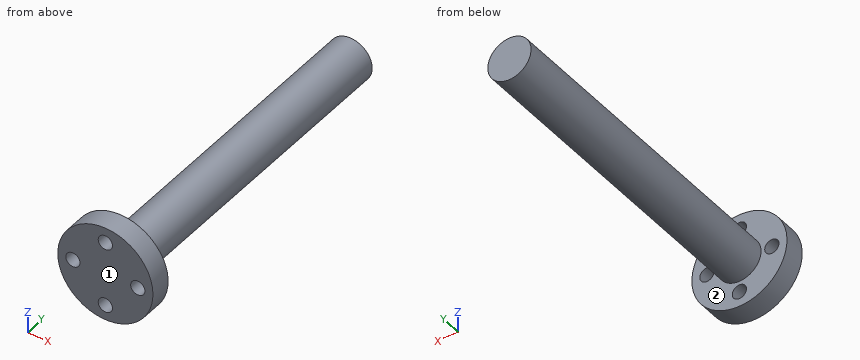
```python
from build123d import *

# Parameters (mm, degrees)
SKETCH1_R                                 = 10
OUTPUT_SHAFT_20MM_DEPTH                   = 161
SKETCH2_R                                 = 22
SKETCH2_R_2                               = 3.3
OUTPUT_LOWER_FLANGE_WITH_BOLT_HOLES_DEPTH = 10


with BuildPart() as part:
    # Sketch1 → Output_Shaft_20mm (new body)
    with BuildSketch(Plane(origin=(0, 0, 0), x_dir=(1, 0, 0), z_dir=(0, 1, 0))):
        with Locations(Location((0, 0, 0), (0, 0, 270))):
            Circle(SKETCH1_R)
    extrude(amount=OUTPUT_SHAFT_20MM_DEPTH)

    # Sketch2 → Output_Lower_Flange_With_Bolt_Holes (add)
    with BuildSketch(Plane(origin=(0, 0, 0), x_dir=(1, 0, 0), z_dir=(0, 1, 0))):
        with Locations(Location((0, 0, 0), (0, 0, 270))):
            Circle(SKETCH2_R)
        with Locations(Location((-15, 0, 0), (0, 0, 270))):
            Circle(SKETCH2_R_2, mode=Mode.SUBTRACT)
        with Locations(Location((15, 0, 0), (0, 0, 270))):
            Circle(SKETCH2_R_2, mode=Mode.SUBTRACT)
        with Locations(Location((0, -15, 0), (0, 0, 270))):
            Circle(SKETCH2_R_2, mode=Mode.SUBTRACT)
        with Locations(Location((0, 15, 0), (0, 0, 270))):
            Circle(SKETCH2_R_2, mode=Mode.SUBTRACT)
    extrude(amount=OUTPUT_LOWER_FLANGE_WITH_BOLT_HOLES_DEPTH)


solid = part.part
```
Check sheet for the modelled part. Datum: model origin and axes. Units: mm. Face numbers are marked on the shaded views. A direction names the side the tool comes from. Coordinates: 2 decimals unless noted, no trailing zeros. Order: outer loops, then holes, each group sorted by start corner. A loop starts at its lowest first (then second) coordinate and runs counter-clockwise, first axis right, second up. Notation, with made-up numbers: (15.25, 38.5) -> (53.25, 38.5) arc R32 cw to (53.25, 67.5) -> close; hole circle Ø4 at (26, 33.25). An arc over 180 degrees is marked (long way). Write each question's results on one line, items separated by ' | '. Start each with the question number.
1) Section check A-A (z = 0). Enter the section's corners in (x, y), and give its area (3 significant figures).
2) Section check C-C (x = 15). Enter the section's corners in (y, z).
3) Section check B-B (z = -15). Enter the section's corners in (x, y), and give its area (3 significant figures).
4) Set-up check for the marked faces 1 and 2: record each of +Z, -Z, +X, -X, +Y, -Y from which the full face is reachable in a straight line by a thin tool's end or side.
5) Material ranges on line 1 along X through (y, z) = (7, 0); line 2 along Y through (x, z) = (-20, -2.5); line 3 along Z through (x, y) = (-4, 41), recorded low to high.
6) Depth check by flat-ended pin: pin 1 (6 mm diameter, centred on x = 0, z = 15, fed in from -Y); pin 2 (1 mm diameter, centred on y = 46, z = 1, fed in from -X); pin 3 (4 mm diameter, centred on x = 6, y = 83.5, fed in from -Z); pin 4 (8.5 mm diameter, centred on x = 0, z = -15, fed in from +Y). Enter the tip coordinate at first touch or a pass-through.
7) Section check D-D (x = 1.5). Enter the section's corners in (y, z), and give its area (3 significant figures).
Checked values:
1) outline: (-22, 0) -> (-18.3, 0) -> (-18.3, 10) -> (-22, 10) -> close; (-11.7, 0) -> (11.7, 0) -> (11.7, 10) -> (10, 10) -> (10, 161) -> (-10, 161) -> (-10, 10) -> (-11.7, 10) -> close; (18.3, 0) -> (22, 0) -> (22, 10) -> (18.3, 10) -> close | area: 3,330 mm²
2) outline: (0, -16.09) -> (10, -16.09) -> (10, -3.3) -> (0, -3.3) -> close; (0, 3.3) -> (10, 3.3) -> (10, 16.09) -> (0, 16.09) -> close
3) outline: (-16.09, 0) -> (-3.3, 0) -> (-3.3, 10) -> (-16.09, 10) -> close; (3.3, 0) -> (16.09, 0) -> (16.09, 10) -> (3.3, 10) -> close | area: 256 mm²
4) face 1: +Z, -Z, +X, -X, -Y | face 2: +Y
5) line 1: -22 to -18.3, -11.7 to 11.7, 18.3 to 22 | line 2: 0 to 10 | line 3: -9.17 to 9.17
6) pin 1: through | pin 2: x = -9.99 | pin 3: z = -9.17 | pin 4: y = 10
7) outline: (0, -21.95) -> (10, -21.95) -> (10, -17.94) -> (0, -17.94) -> close; (0, -12.06) -> (10, -12.06) -> (10, -9.89) -> (161, -9.89) -> (161, 9.89) -> (10, 9.89) -> (10, 12.06) -> (0, 12.06) -> close; (0, 17.94) -> (10, 17.94) -> (10, 21.95) -> (0, 21.95) -> close | area: 3,310 mm²
